Geometry check sheet. Reference: the model listing, model coordinates, mm. Face numbers are marked on the shaded views. A direction names the side the tool comes from. Coordinates: 2 decimals unless noted, no trailing zeros. Order: outer loops, then holes, each group sorted by start corner. A loop starts at its lowest first (then second) coordinate and runs counter-clockwise, first axis right, second up. Notation, with made-up numbers: (-23, -6.5) - (23, -6.5) arc R20 ccw to (23, 26.5) - close; hole circle Ø10 at (-16.75, 63.25). An arc over 180 degrees is marked (long way). Use CSV: the item, a comma, the result in double quotes. Start each with the question number.
1) Sectioned sample at A-A, the plane x = -17. Record the cut outline in (y, z).
2) Tool access check on the marked faces 1, 2 and 3. Record the directions out of +Z, -Z, +X, -X, +Y, -Y that give a thin tool (end or side, any length) a straight path to the whole face; none if there is none.
3) Depth check by flat-ended pin: P1, Ø1, axis at x = -45, y = -7, coming from the -Z side; P2, Ø5, axis at y = -12, z = -0.5, coming from the +X side; P3, Ø6, axis at y = -14, z = -3, coming from the -X side. Enter the tip coordinate at first touch or a pass-through.
4) Sectioned sample at B-B, the plane y = -12. Record the cut outline in (x, z).
5) Sectioned sample at D-D, the plane z = 2. Record the cut outline in (x, y).
6) Sectioned sample at C-C, the plane x = -32. Record the cut outline in (y, z), and give its area (3 significant figures).
7) Thickness scan on probe 1 along X at (y, z) = (-11, -24); probe 2 along Z at (x, y) = (-31.5, -7.5); probe 3 along Z at (x, y) = (-32.5, -5). Record the ranges inside material, lowest first. Write a range as [from, to].
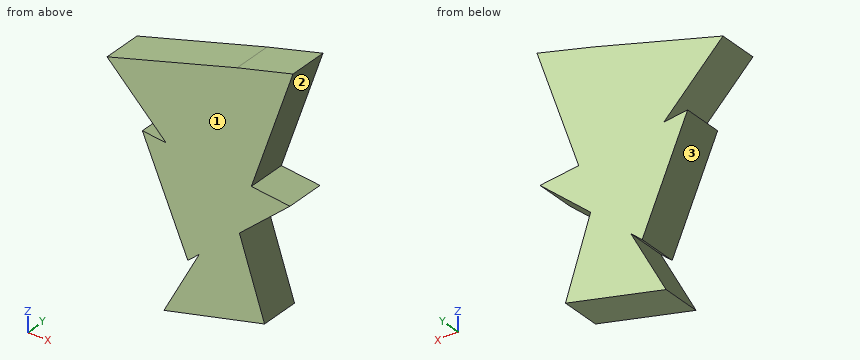
from build123d import *

# Parameters (mm, degrees)
F1_DEPTH = 20


with BuildPart() as f1:
    # F0 (on Front) → F1 (new body)
    with BuildSketch(Plane.XZ):
        Polygon((0, -4.78173), (-16.802281, 16.61918), (-25.650827, 25.3713), (-37.688062, 26.623173), (-14.656468, -26.31958), (-8.858471, -21.258901), align=None)
        Polygon((-25.650827, 25.3713), (-16.802281, 16.61918), (0, -4.78173), (-8.858471, -21.258901), (11.46337, -3.52134), (10.295821, 0), (17.490609, 20.884591), align=None)
        Polygon((-55.597428, 54.991562), (-25.650827, 25.3713), (17.490609, 20.884591), (38.609326, 82.186714), (10.295821, 74.528098), align=None)
        Polygon((37.08984, 18.846272), (17.490609, 20.884591), (10.295821, 0), (11.46337, -3.52134), align=None)
        Polygon((11.46337, -3.52134), (-8.858471, -21.258901), (-26.769133, -54.573569), (24.195176, -41.920602), align=None)
    extrude(amount=F1_DEPTH)


solid = f1.part
Evaluation:
1,outline,"(-20, -52.15) - (0, -52.15) - (0, -36.4) - (-20, -36.4) - close; (-20, -20.93) - (0, -20.93) - (0, 66.44) - (-20, 66.44) - close"
2,face 1,"+Z, -Z, +X, -X, -Y"
2,face 2,"+X, +Y, -Y"
2,face 3,"-X, +Y, -Y"
3,P1,"z = 44.02"
3,P2,"x = 17.79"
3,P3,"x = -26.11"
4,outline,"(-55.6, 54.99) - (-25.65, 25.37) - (-37.69, 26.62) - (-14.66, -26.32) - (-8.86, -21.26) - (-26.77, -54.57) - (24.2, -41.92) - (11.46, -3.52) - (37.09, 18.85) - (17.49, 20.88) - (38.61, 82.19) - (10.3, 74.53) - close"
5,outline,"(-26.98, -20) - (17.79, -20) - (17.79, 0) - (-26.98, 0) - close"
6,outline,"(-20, 13.55) - (0, 13.55) - (0, 26.03) - (-20, 26.03) - close; (-20, 31.65) - (0, 31.65) - (0, 61.99) - (-20, 61.99) - close"
6,area,"856 mm²"
7,probe 1,"[-15.67, -12], [-10.33, 18.25]"
7,probe 2,"[12.4, 25.98], [31.16, 62.14]"
7,probe 3,"[14.7, 26.08], [32.15, 61.84]"
